```python
from build123d import *

# Parameters (mm, degrees)
SKETCH2_W           = 19.1
SKETCH2_H           = 13
BOSS_EXTRUDE1_DEPTH = 2
BOSS_EXTRUDE2_DEPTH = 2
SKETCH4_R           = 0.8
BOSS_EXTRUDE3_DEPTH = 1.5
BOSS_EXTRUDE3_TAPER = 5
SKETCH5_W           = 9
SKETCH5_H           = 2
CUT_EXTRUDE1_DEPTH  = 2


with BuildPart() as part:
    # Sketch2 → Boss-Extrude1 (new body)
    with BuildSketch(Plane(origin=(0, 0, 0), x_dir=(1, 0, 0), z_dir=(0, 1, 0))):
        Rectangle(SKETCH2_W, SKETCH2_H)
    extrude(amount=BOSS_EXTRUDE1_DEPTH)

    # Sketch3 → Boss-Extrude2 (add)
    with BuildSketch(Plane.ZY.offset(9.55)):
        with BuildLine():
            Line((6.5, 0), (6.5, 23))
            Line((6.5, 23), (1.5, 23))
            ThreePointArc((1.5, 23), (-4.156854249, 20.656854249), (-6.5, 15))
            Line((-6.5, 15), (-6.5, 0))
            Line((-6.5, 0), (6.5, 0))
        make_face()
    boss_extrude2 = extrude(amount=BOSS_EXTRUDE2_DEPTH)

    # Sketch4 → Boss-Extrude3 (add)
    with BuildSketch(Plane(origin=(-9.55, 0, 0), x_dir=(0, 0, -1), z_dir=(1, 0, 0))):
        with Locations((0, 18)):
            Circle(SKETCH4_R)
    boss_extrude3 = extrude(amount=BOSS_EXTRUDE3_DEPTH, taper=BOSS_EXTRUDE3_TAPER)

    # Sketch5 → Cut-Extrude1 (cut)
    with BuildSketch(Plane(origin=(-9.55, 0, 0), x_dir=(0, 0, -1), z_dir=(1, 0, 0))):
        with Locations((0, 3)):
            Rectangle(SKETCH5_W, SKETCH5_H)
    cut_extrude1 = extrude(amount=-CUT_EXTRUDE1_DEPTH, mode=Mode.SUBTRACT)

    # Mirror1: Boss-Extrude2, Boss-Extrude3, Cut-Extrude1 across plane
    add(boss_extrude2.mirror(Plane(origin=(0, 0, 0), x_dir=(0, 0, 1), z_dir=(1, 0, 0))))
    add(boss_extrude3.mirror(Plane(origin=(0, 0, 0), x_dir=(0, 0, 1), z_dir=(1, 0, 0))))
    add(cut_extrude1.mirror(Plane(origin=(0, 0, 0), x_dir=(0, 0, 1), z_dir=(1, 0, 0))), mode=Mode.SUBTRACT)


solid = part.part
```
Could you check a few things on this model? Use its own coordinates, in mm. A direction names the side the tool comes from. Give positions to 0.01 mm unless a question says otherwise; leave off trailing zeros. Order: outer loops, then holes, each group sorted by start corner. A loop starts at its lowest first (then second) coordinate and runs counter-clockwise, first axis right, second up.
Q1. Suppose I cut it at C-C, the plane z = 0. Write out the boundary of the cut face in (x, y), and give its area (3 significant figures).
Q2. We'd pull the mould along Y, two halves only. Please class faces 1 (the flat face through (-11, 3, -4.5)), 2 (the flat face through (8.05, 18, 0)), 3 (the cylindrical face through (-10.536, 20.719, -4.094)): +Y half, -Y half, draft (parallel to the pull), parting line (faces both ways), or undercut.
Q3. For faces 4 (the flat face through (11, 4, 0)), 5 (the flat face through (11.55, 12, 0)), 6 (the flat face through (-8.05, 18, 0)), 7 (the flat face through (11, 23, 4)), 8 (the conical face through (8.79, 17.284, 0.159)), which set-ups out of +Z, -Z, +X, -X, +Y, -Y let a thin tool reach every point of the face, with its end or its side?
Q4. Suppose I cut it at A-A, the plane y = 7.25. Write out the boundary of the cut face in (x, z), and give its area (3 significant figures).
Q5. I'm going to push flat-ended pins straight in: P1, Ø1, axis at x = 11, z = 1, coming from the -Y side; P2, Ø4, axis at x = -4, z = 3, coming from the +Y side. Where does each tip first touch, or does it pass through?
Q6. Suppose I cut it at B-B, the plane z = 2. Write out the boundary of the cut face in (x, y), and give its area (3 significant figures).
Q7. Suppose I cut it at D-D, the plane x = -0.25. Write out the boundary of the cut face in (y, z).
Q8. If I drill on line 1 along X through (y, z) = (19, -3); line 2 along Y through (x, z) = (-6, -5); line 3 along Z through (x, y) = (9, 17.5), over which ranges is the centre line in solid material (lowest first)?
Solution:
1. outline: (-11.55, 0) - (11.55, 0) - (11.55, 2) - (-11.55, 2) - close; (-11.55, 4) - (-9.55, 4) - (-9.55, 17.2) - (-8.05, 17.33) - (-8.05, 18.67) - (-9.55, 18.8) - (-9.55, 22.86) - (-11.55, 22.86) - close; (8.05, 17.33) - (9.55, 17.2) - (9.55, 4) - (11.55, 4) - (11.55, 22.86) - (9.55, 22.86) - (9.55, 18.8) - (8.05, 18.67) - close
1. area: 126 mm2
2. face 1: undercut
2. face 2: draft
2. face 3: +Y half
3. face 4: +X, -X
3. face 5: +Z, -Z, +X, +Y, -Y
3. face 6: +Z, -Z, +Y
3. face 7: +Z, -Z, +X, -X, +Y
3. face 8: none
4. outline: (-11.55, -6.5) - (-9.55, -6.5) - (-9.55, 6.5) - (-11.55, 6.5) - close; (9.55, -6.5) - (11.55, -6.5) - (11.55, 6.5) - (9.55, 6.5) - close
4. area: 52.0 mm2
5. P1: stops at y = 0
5. P2: stops at y = 2
6. outline: (-11.55, 0) - (11.55, 0) - (11.55, 2) - (-11.55, 2) - close; (-11.55, 4) - (-9.55, 4) - (-9.55, 23) - (-11.55, 23) - close; (9.55, 4) - (11.55, 4) - (11.55, 23) - (9.55, 23) - close
6. area: 122 mm2
7. outline: (0, -6.5) - (2, -6.5) - (2, 6.5) - (0, 6.5) - close
8. line 1: x = -11.55 to -9.55, 9.55 to 11.55
8. line 2: y = 0 to 2
8. line 3: z = -0.56 to 0.56
